Verification items for the finished model (mm, model axes). A direction names the side the tool comes from. Coordinates: 2 decimals unless noted, no trailing zeros. Order: outer loops, then holes, each group sorted by start corner. A loop starts at its lowest first (then second) coordinate and runs counter-clockwise, first axis right, second up. Notation, with made-up numbers: (81.5, 10.25) -> (121.5, 10.25) arc R24 ccw to (121.5, 23.25) -> close; hole circle Ø11 at (-8, -32). An arc over 180 degrees is marked (long way). Write each question's results on one line, items separated by ' | '. Start each with the question number.
(1) Thickness scan on probe 1 along X at (y, z) = (0.85, -15.7); probe 2 along Y at (x, z) = (-63, -18); probe 3 along Z at (x, y) = (-20, 25). Record the ranges inside material, lowest first. Write a range as [from, to].
(2) Cross-section at C-C on y = 21. Enter the section's corners in (x, z).
(3) Set-up check for faces 1 (the flat face through (-77.8, 2, -25)), 2 (the flat face through (-25, 23, -25)), 3 (the flat face through (-10, 5, 1)): record each of +Z, -Z, +X, -X, +Y, -Y from which the full face is reachable in a straight line by a thin tool's end or side.
(4) Cross-section at A-A on z = -15.7. Enter the section's corners in (x, y).
(5) Draft check along Y on faces 4 (the flat face through (-50, 24, -3)), 5 (the cylindrical face through (-4.764, 5.724, 0.986)), 6 (the cylindrical face through (-14.236, 5.724, 0.986)). Enter one of: +Y half, -Y half, draft (parallel to the pull), parting line (faces both ways), or undercut.
(6) Cross-section at B-B on x = -39.7. Enter the section's corners in (y, z), and give its area (3 significant figures).
(7) Cross-section at D-D on x = -31. Enter the section's corners in (y, z), and give its area (3 significant figures).
(8) Go/stop test with flat-tipped pins: pin 1 (0.7 mm diameter, centred on y = 38.5, z = 0.5, fed in from -X); pin 2 (15 mm diameter, centred on x = -60, z = -28.5, fed in from +Y); pin 3 (12 mm diameter, centred on y = 12.5, z = -7.5, fed in from +X). Record where each tip stops, or that it passes through.
```python
from build123d import *

# Parameters (mm, degrees)
SKETCH1_W           = 25
SKETCH1_H           = 45
BOSS_EXTRUDE1_DEPTH = 2
SKETCH2_W           = 11
SKETCH2_H           = 6.5
CUT_EXTRUDE1_DEPTH  = 19.78
FILLET1_R           = 2.54
BOSS_EXTRUDE2_DEPTH = 2
SKETCH4_W           = 52.8
SKETCH4_H           = 3
BOSS_EXTRUDE3_DEPTH = 50.8
BOSS_EXTRUDE4_DEPTH = 5
SKETCH7_R           = 6.35
CUT_EXTRUDE3_DEPTH  = 5


with BuildPart() as part:
    # Sketch1 → Boss-Extrude1 (new body)
    with BuildSketch(Plane.XY):
        with Locations((-12.5, 22.5)):
            Rectangle(SKETCH1_W, SKETCH1_H)
    extrude(amount=BOSS_EXTRUDE1_DEPTH)

    # Sketch2 → Cut-Extrude1 (cut)
    with BuildSketch(Plane.XY.offset(2)):
        with Locations((-9.5, 8.25)):
            Rectangle(SKETCH2_W, SKETCH2_H)
        with Locations((-9.5, 38.75)):
            Rectangle(SKETCH2_W, SKETCH2_H)
    extrude(amount=-CUT_EXTRUDE1_DEPTH, mode=Mode.SUBTRACT)

    # Fillet1
    fillet1_edges = [part.edges().sort_by_distance(p)[0] for p in [
        (-15, 11.5, 1),
        (-4, 11.5, 1),
        (-4, 5, 1),
        (-15, 5, 1),
        (-15, 42, 1),
        (-4, 42, 1),
        (-4, 35.5, 1),
        (-15, 35.5, 1),
    ]]
    fillet(fillet1_edges, radius=FILLET1_R)

    # Sketch3 → Boss-Extrude2 (add)
    with BuildSketch(Plane.ZY.offset(25)):
        Polygon((2, 0), (0, 0), (-50.8, 0), (-50.8, 45), (0, 45), (2, 45), align=None)
    extrude(amount=BOSS_EXTRUDE2_DEPTH)

    # Sketch4 → Boss-Extrude3 (add)
    with BuildSketch(Plane.ZY.offset(27)):
        with Locations((-24.4, 1.5)):
            Rectangle(SKETCH4_W, SKETCH4_H)
    extrude(amount=BOSS_EXTRUDE3_DEPTH)

    # Sketch5 → Boss-Extrude4 (add)
    with BuildSketch(Plane.XY.offset(2)):
        Polygon((-77.8, 3), (-27, 45), (-27, 42.151802073), (-77.8, 0), align=None)
    extrude(amount=-BOSS_EXTRUDE4_DEPTH)

    # Sketch7 → Cut-Extrude3 (cut)
    with BuildSketch(Plane(origin=(0, 3, 0), x_dir=(1, 0, 0), z_dir=(0, 1, 0))):
        with Locations(Location((-39.7, 15.7, 0), (0, 0, 270))):
            Circle(SKETCH7_R)
    extrude(amount=-CUT_EXTRUDE3_DEPTH, mode=Mode.SUBTRACT)


solid = part.part
```
Results are:
1) probe 1: x = [-77.8, -46.05], [-33.35, -25] | probe 2: y = [0, 3] | probe 3: z = [0, 2]
2) outline: (-56.03, -3) -> (-52.49, -3) -> (-52.49, 2) -> (-56.03, 2) -> close; (-27, -50.8) -> (-25, -50.8) -> (-25, 0) -> (0, 0) -> (0, 2) -> (-27, 2) -> close
3) face 1: +Z, -Z, -X, +Y, -Y | face 2: -Z, +X, +Y, -Y | face 3: +Z, -Z
4) outline: (-77.8, 0) -> (-46.05, 0) -> (-46.05, 3) -> (-77.8, 3) -> close; (-33.35, 0) -> (-25, 0) -> (-25, 45) -> (-27, 45) -> (-27, 3) -> (-33.35, 3) -> close
5) face 4: draft | face 5: undercut | face 6: undercut
6) outline: (0, -50.8) -> (3, -50.8) -> (3, -22.05) -> (0, -22.05) -> close; (0, -9.35) -> (3, -9.35) -> (3, 2) -> (0, 2) -> close; (31.61, -3) -> (34.5, -3) -> (34.5, 2) -> (31.61, 2) -> close | area: 135 mm2
7) outline: (0, -50.8) -> (3, -50.8) -> (3, 2) -> (0, 2) -> close; (38.83, -3) -> (41.69, -3) -> (41.69, 2) -> (38.83, 2) -> close | area: 173 mm2
8) pin 1: stops at x = -35.29 | pin 2: stops at y = 3 | pin 3: stops at x = -25
